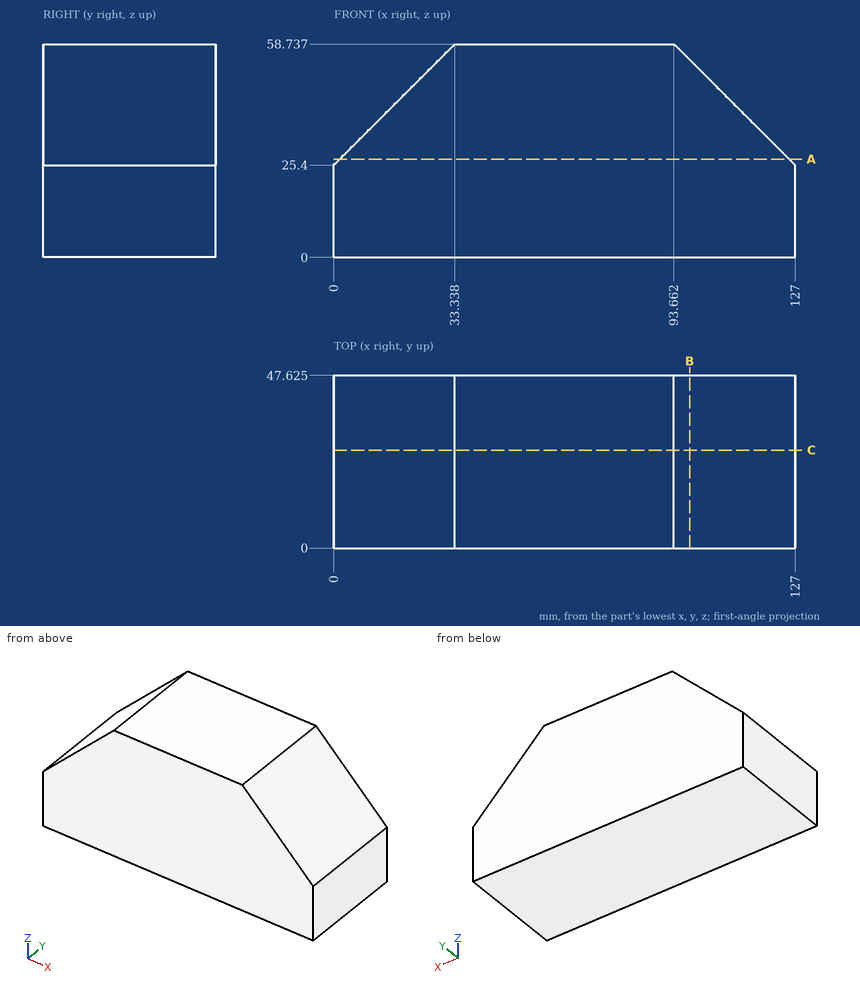
Design review of the part shown in the three views and the two pictorial views. Dimensions are in mm from the part's minimum x, y and z. Coordinates: 2 decimals unless noted, no trailing zeros. Order: outer loops, then holes, each group sorted by start corner. A loop starts at its lowest first (then second) coordinate and runs counter-clockwise, first axis right, second up.
Item 1: Take a section at B-B, the plane x = 98. Write out the cut boundary in (y, z) (1 decimal).
Item 2: For line 1 (X direction, y = 8, z = 49.5); line 2 (Z direction, x = 6, y = 40); line 3 (Z direction, x = 110, y = 23), list the stretches that pass through material, from the lowest coordinate up.
Item 3: For pin 1 Ø5 at (y, z) = (23.5, 47.5) entering from +X; pin 2 Ø4 at (y, z) = (6.5, 28.5) entering from -X; pin 3 Ø12 at (y, z) = (34.5, 36) entering from +X, all flat-tipped, find the tip position at first contact; note any pin that passes through.
Item 4: Take a section at A-A, the plane z = 27. Write out the cut boundary in (x, y) (1 decimal).
Item 5: Take a section at C-C, the plane y = 27. Write out the cut boundary in (x, z), then the cut area to 3 significant figures.
The answers:
1. outline: (0, 0) - (47.6, 0) - (47.6, 54.4) - (0, 54.4) - close
2. line 1: x = 24.1 to 102.9
2. line 2: z = 0 to 31.4
2. line 3: z = 0 to 42.4
3. pin 1: stops at x = 107.4
3. pin 2: stops at x = 1.1
3. pin 3: stops at x = 122.4
4. outline: (1.6, 0) - (125.4, 0) - (125.4, 47.6) - (1.6, 47.6) - close
5. outline: (0, 0) - (127, 0) - (127, 25.4) - (93.66, 58.74) - (33.34, 58.74) - (0, 25.4) - close
5. area: 6,350 mm2
